For this review, use the dimensioned drawing (mm, ordinates from the lowest corner) and the shaded views. Coordinates: 2 decimals unless noted, no trailing zeros. One line per question, with ' | ' between items. Start each with the question number.
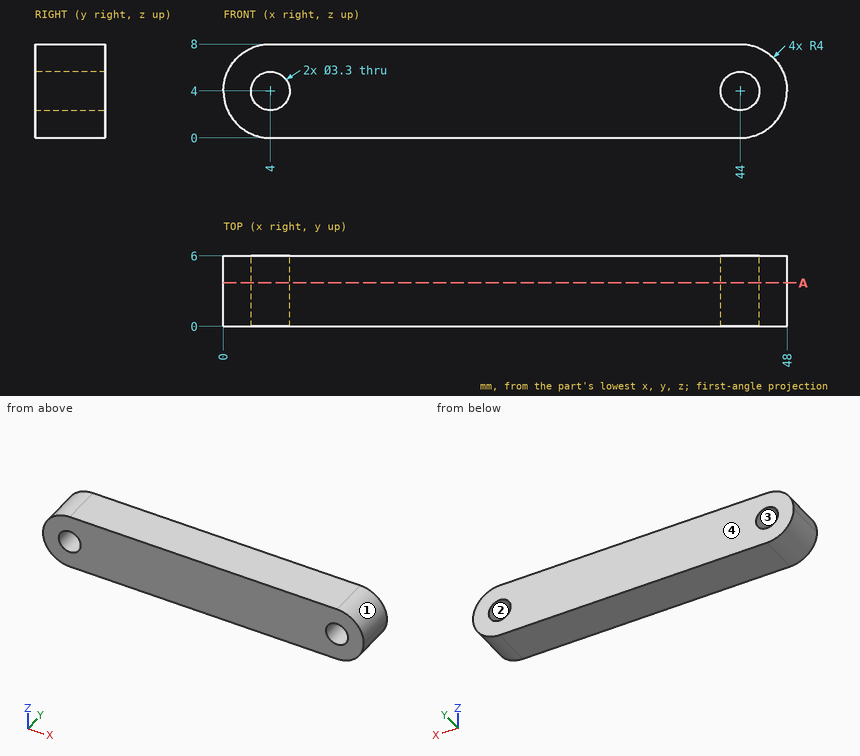
1) Wall thickness on L1, parallel to X at y = 1.85, z = 4; L2, parallel to X at y = 2.4, z = 3; L3, parallel to Z at x = 3.5, y = 0.65: over which ranges is each line inside the solid? List them lowest first.
2) Insertion check: pin 1 Ø1.5 at (x, z) = (6, 5) entering from -Y. The pin has a flat end and moves straight along its axis. Give the tip position at first contact, or say it passes through.
3) Consider section A-A, the plane y = 3.7. Give the number of separate pieces and of enclosed holes in the cut face, plus the area to 3 significant figures.
4) Mouldability with a two-part tool opening along X and no side actions: class the marked faces 1, 2, 3 and 4 as +X half, -X half, draft (parallel to the pull), parting line (faces both ways), or undercut.
Filled sheet:
1) L1: 0 to 2.35, 5.65 to 42.35, 45.65 to 48 | L2: 0.13 to 2.69, 5.31 to 42.69, 45.31 to 47.87 | L3: 0.03 to 2.43, 5.57 to 7.97
2) pin 1: y = 0
3) separate pieces: 1 | enclosed holes: 2 | area: 353 mm^2
4) face 1: +X half | face 2: undercut | face 3: undercut | face 4: draft
